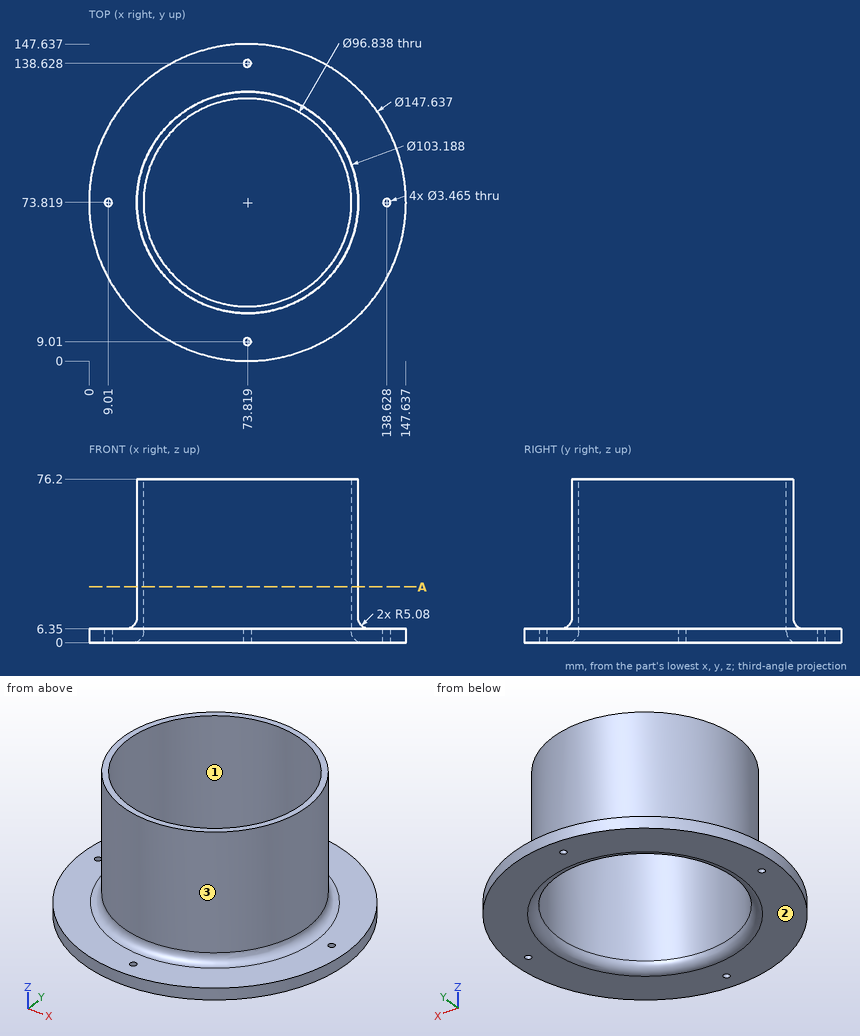
Source: three-view drawing plus pictorial views. Frame: mm from the lowest corner of the part. Coordinates: 2 decimals unless noted, no trailing zeros. Order: outer loops, then holes, each group sorted by start corner. A loop starts at its lowest first (then second) coordinate and runs counter-clockwise, first axis right, second up.
Item 1: Material intervals for line 1 (Z direction, x = 28.5, y = 131); line 2 (Y direction, x = 95.5, z = 73.5) (1 decimal); line 3 (Y direction, x = 71, z = 24) (1 decimal), sorted ascending.
Output values:
line 1: z = 0 to 6.35
line 2: y = 27 to 30.5, 117.1 to 120.6
line 3: y = 22.3 to 25.5, 122.2 to 125.3
Item 2: Cut plane A-A (z = 26). Return loops of the section in (x, y).
Output values:
outline: circle Ø103.19 at (73.82, 73.82); hole circle Ø96.84 at (73.82, 73.82)
Item 3: First-contact query: P1, Ø2, axis at x = 92.5, z = 9.5, coming from the +Y side; P2, Ø8, axis at x = 127, y = 110, coming from the +Z side; P3, Ø1.5, axis at x = 52.5, z = 53.5, coming from the -Y side. Flat tips, straight axial feed; report the tip coordinate or a pass-through.
Output values:
P1: stops at y = 123
P2: stops at z = 6.35
P3: stops at y = 26.5
Item 4: Pull-direction query (Y, two-part tool) for the marked faces 1, 2 and 3; classes: pulls with the +Y half, pulls with the -Y half, needs draft (parallel to the pull), parting line crosses it, or undercut.
Output values:
face 1: undercut
face 2: needs draft
face 3: parting line crosses it
